from build123d import *

# Parameters (mm, degrees)
F0_R     = 0.9
F0_W     = 19
F0_H     = 3
F1_DEPTH = 2
F2_R     = 0.89999
F3_R     = 0.8


# Not quite as in the source:
# - a fillet or chamfer is up to 0.001 mm smaller than in the source, because OpenCascade refuses the exact size


with BuildPart() as f1:
    # F0 (on Top) → F1 (new body)
    with BuildSketch(Plane.XY):
        with BuildLine():
            Line((12.5, 7.5), (-12.5, 7.5))
            Line((-12.5, 7.5), (-12.5, -7.5))
            Line((-12.5, -7.5), (-2.5, -7.5))
            Line((-2.5, -7.5), (-2.5, -8.4))
            ThreePointArc((-2.5, -8.4), (0, -10.9), (2.5, -8.4))
            Line((2.5, -8.4), (2.5, -7.5))
            Line((2.5, -7.5), (12.5, -7.5))
            Line((12.5, -7.5), (12.5, 7.5))
        make_face()
        with Locations((0, -8.4)):
            Circle(F0_R, mode=Mode.SUBTRACT)
        with Locations((0, -3)):
            Rectangle(F0_W, F0_H, mode=Mode.SUBTRACT)
        with Locations((0, 3)):
            Rectangle(F0_W, F0_H, mode=Mode.SUBTRACT)
    extrude(amount=F1_DEPTH)

    # F2 (radius 0.9 in the source; OpenCascade refuses exactly that, so slightly less here)
    f2_edges = [f1.edges().sort_by_distance(p)[0] for p in [
        (2.5, -7.5, 1),
        (-2.5, -7.5, 1),
    ]]
    fillet(f2_edges, radius=F2_R)

    # F3
    f3_edges = [f1.edges().sort_by_distance(p)[0] for p in [
        (12.5, 0, 2),
        (7.949995, -7.5, 2),
        (-12.5, 0, 2),
        (0, 7.5, 2),
    ]]
    fillet(f3_edges, radius=F3_R)


solid = f1.part
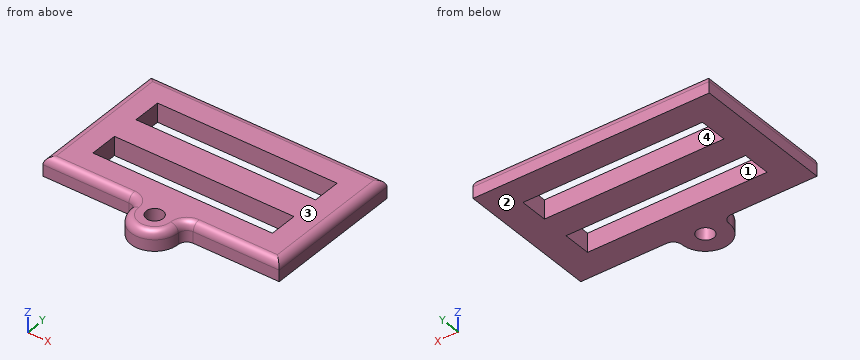
Build history of the part. All positions in model axes, mm. Face numbers are marked on the shaded views. A direction names the side the tool comes from. Give positions to 0.01 mm unless a question says otherwise; leave off trailing zeros. Order: outer loops, then holes, each group sorted by start corner. A loop starts at its lowest first (then second) coordinate and runs counter-clockwise, first axis right, second up. Notation, with made-up numbers: M 36,89 L 70,89 A9 ccw 70,102 Z; hole C 15,53.25 d10. An arc over 180 degrees is marked long. Use one line per item in the form item = value.
Q1. Slice it at A-A, the plane x = 0. Write the cut outline in (y, z).
Conclusion:
outline = M -10.9,0 L -9.3,0 L -9.3,2 L -10.1,2 A0.8 ccw -10.9,1.2 Z; M -7.5,0 L -4.5,0 L -4.5,2 L -7.5,2 Z; M -1.5,0 L 1.5,0 L 1.5,2 L -1.5,2 Z; M 4.5,0 L 7.5,0 L 7.5,1.2 A0.8 ccw 6.7,2 L 4.5,2 Z
Q2. Slice it at D-D, the plane x = 9. Write the cut outline in (y, z).
Conclusion:
outline = M -7.5,0 L -4.5,0 L -4.5,2 L -6.7,2 A0.8 ccw -7.5,1.2 Z; M -1.5,0 L 1.5,0 L 1.5,2 L -1.5,2 Z; M 4.5,0 L 7.5,0 L 7.5,1.2 A0.8 ccw 6.7,2 L 4.5,2 Z
Q3. Slice it at B-B, the plane z = 0.6. State how many separate pieces and enclosed holes the cut face has, and give its area (3 significant figures).
Conclusion:
separate_pieces = 1
enclosed_holes = 3
area = 273 mm2
Q4. Pin check, flat tips, straight feed: P1, Ø0.6, axis at x = 7.5, z = 0.5, coming from the -Y side; P2, Ø1.1, axis at x = 0, y = -8.4, coming from the -Z side; P3, Ø1, axis at x = -2, z = 1.5, coming from the -Y side. Stop position of each tip, or through.
Conclusion:
P1 = -7.5
P2 = through
P3 = -10.36
Q5. Wall check: probe 1 along Y at (x, z) = (-6, 0.45); probe 2 along Y at (x, z) = (0, 0.8); probe 3 along Y at (x, z) = (-4, 1.75). Give the ranges that are in metal, low to high.
Conclusion:
probe_1 = -7.5 to -4.5, -1.5 to 1.5, 4.5 to 7.5
probe_2 = -10.9 to -9.3, -7.5 to -4.5, -1.5 to 1.5, 4.5 to 7.5
probe_3 = -7.28 to -4.5, -1.5 to 1.5, 4.5 to 7.28
Q6. Which spindle directions (+Z, -Z, +X, -X, +Y, -Y) get a long thin tool onto all of the face, cutting with end or side? Do the marked faces 3 and 4. Say none if no direction does.
Conclusion:
face_3 = +Z, +X, -X, +Y, -Y
face_4 = +Z, -Z
Q7. Pull direction X, two halves, no side cores. Call the marked faces 1 and 2: released by +X, released by -X, zero draft, split by the parting line, or undercut.
Conclusion:
face_1 = undercut
face_2 = zero draft
Q8. Slice it at C-C, the plane y = 3.5. Write the cut outline in (x, z).
Conclusion:
outline = M -12.5,0 L -9.5,0 L -9.5,2 L -11.7,2 A0.8 ccw -12.5,1.2 Z; M 9.5,0 L 12.5,0 L 12.5,1.2 A0.8 ccw 11.7,2 L 9.5,2 Z
